Part model, mm, in its own coordinate system. A direction names the side the tool comes from. Coordinates: 2 decimals unless noted, no trailing zeros. Loops run counter-clockwise (first coordinate to the right, second up) from the corner with the lowest first, then second, coordinate; pieces in that order, holes last. Notation, with made-up numbers: (86, 78) -> (104, 78) arc R19 ccw to (104, 96) -> close; hole circle Ø4 at (80, 89). An arc over 180 degrees is marked (long way). Use one line per item in the form item = value. Start each with the question number.
(1) Pin check, flat tips, straight feed: P1, Ø5, axis at y = 5, z = -50, coming from the +X side; P2, Ø5, axis at y = 5.5, z = -41, coming from the -X side; P3, Ø2.5, axis at x = 0, z = 0.5, coming from the -Y side; P4, Ø2.5, axis at x = -17, z = 0, coming from the +Y side. Stop position of each tip, or through.
(2) Band-saw the part on A-A on x = 48. Give the cut face in (y, z), then the cut area to 3 significant figures.
(3) Mould opens along X. For faces 1 (the flat face through (-1, 9, 1)), 2 (the flat face through (-35.275, 3.042, -20.366)), 3 (the cylindrical face through (-0.652, 3.042, 5.964)) say: +X half, -X half, draft (parallel to the pull), parting line (faces both ways), or undercut.
(4) Drill centre lines: L1, parallel to X at y = 7.2, z = 0; L2, parallel to Y at x = -30, z = -43. Where is each one in solid material? Low to high. Write a range as [from, to].
(5) Band-saw the part on B-B on z = 24. Give the cut face in (x, y).
(6) 3-axis set-ups, long thin cutter, end or side, ignore diameter. For faces 4 (the flat face through (33.263, 3.042, 24.176)), 5 (the flat face through (-24.176, 3.042, 33.263)), 6 (the cylindrical face through (5.964, 3.042, 0.652)), 7 (the cylindrical face through (0.652, 3.042, -5.964)), 8 (the flat face through (0, 6, 0)): which of +Z, -Z, +X, -X, +Y, -Y reach the whole face in a straight line?
Autodesk Inventor part; units mm, degrees
ref_plane "YZ Plane" through (0, 0, 0) normal (1, 0, 0) x (0, 1, 0)
ref_plane "XZ Plane" through (0, 0, 0) normal (0, 1, 0) x (-1, 0, 0)
ref_plane "XY Plane" through (0, 0, 0) normal (0, 0, 1) x (1, 0, 0)
sketch "Sketch1" plane through (0, 0, 0) normal (0, 0, 1) x (1, 0, 0)
  line L0 (4, 0) -> (6, 0)
  line L1 (6, 0) -> (6, 6)
  line L2 (6, 6) -> (76.45, 6)
  line L3 (76.45, 6) -> (76.45, 9)
  line L4 (4, 6) -> (4, 0)
  line L5 (0, 9) -> (0, 6)
  line L6 (0, 6) -> (4, 6)
  line L7 (0, 9) -> (13.95, 9)
  line L8 (13.95, 9) -> (13.95, 9)
  line L9 (13.95, 9) -> (16.45, 9)
  line L10 (16.45, 9) -> (16.45, 9)
  line L11 (16.45, 9) -> (76.45, 9)
  point P0 (0, 0)
  dimension "d0" = 4
  dimension "d1" = 6
  dimension "d2" = 0
  dimension "d3" = 3
  dimension "d4" = 2
  dimension "d7" = 2.5
  dimension "d8" = 60
  dimension "d9" = 13.95
  dimension "d10" = 0
revolve "Revolution1" add sketch "Sketch1" angle 360 about axis through (0, 9, 0) along (0, -1, 0)
thread "Thread1"
sketch "Sketch2" plane through (0, 9, 0) normal (0, 1, 0) x (1, 0, 0)
  circle A0 centre (17, 0) radius 1.6
  circle A1 centre (-17, 0) radius 1.6
  circle A2 centre (0, 17) radius 1.6
  circle A3 centre (0, -17) radius 1.6
  point P0 (0, 0)
  dimension "d14" = 3.2
  dimension "d15" = 3.2
  dimension "d16" = 3.2
  dimension "d17" = 3.2
  dimension "d18" = 34
  dimension "d19" = 17
  dimension "d20" = 34
  dimension "d21" = 17
extrude "Extrusion1" cut sketch "Sketch2" against normal through all
sketch "Sketch5" plane through (0, 6, 0) normal (0, -1, 0) x (1, 0, 0)
  circle A0 centre (0, 0) radius 76.45
  circle A1 centre (0, 0) radius 6
  circle A2 centre (0, 0) radius 4
  line L0 (-5.1962, -3) -> (-66.2076, -38.225)
  line L1 (-63.7866, -42.1411) -> (-1.873, -5.7002)
  line L2 (42.1411, -63.7866) -> (5.7002, -1.873)
  line L3 (3, -5.1962) -> (38.225, -66.2076)
  line L4 (63.7866, 42.1411) -> (1.873, 5.7002)
  line L5 (5.1962, 3) -> (66.2076, 38.225)
  line L6 (-42.1411, 63.7866) -> (-5.7002, 1.873)
  line L7 (-3, 5.1962) -> (-38.225, 66.2076)
  arc A3 (38.225, -66.2076) -> (42.1411, -63.7866) centre (0, 0) ccw
  arc A4 (66.2076, 38.225) -> (63.7866, 42.1411) centre (0, 0) ccw
  arc A5 (-38.225, 66.2076) -> (-42.1411, 63.7866) centre (0, 0) ccw
  arc A6 (-66.2076, -38.225) -> (-63.7866, -42.1411) centre (0, 0) ccw
  arc A7 (-5.1962, -3) -> (-1.873, -5.7002) centre (0, 0) ccw
  arc A8 (-3, 5.1962) -> (-5.7002, 1.873) centre (0, 0) ccw
  arc A9 (3, -5.1962) -> (5.7002, -1.873) centre (0, 0) ccw
  arc A10 (5.1962, 3) -> (1.873, 5.7002) centre (0, 0) ccw
  point P0 (0, 0)
  point P1 (-38.225, 66.2076)
  point P2 (-42.1411, 63.7866)
  point P3 (-5.7002, 1.873)
  point P4 (5.1962, 3)
  point P5 (66.2076, 38.225)
  point P6 (63.7866, 42.1411)
  point P7 (1.873, 5.7002)
  point P8 (38.225, -66.2076)
  point P9 (42.1411, -63.7866)
  point P10 (5.7002, -1.873)
  dimension "d35" = 360
extrude "Extrusion3" add sketch "Sketch5" along normal blind 6 contours L5 A1 L4 A0 | A0 L3 A1 L2 | L7 A1 L6 A0 | A0 L0 A1 L1
properties part number "motor platform reaction wheel" material "ABS Plastic"
A:
q1.P1 = 59.74
q1.P2 = -66.05
q1.P3 = 6
q1.P4 = through
q2.outline = (0, 27.71) -> (6, 27.71) -> (6, -59.5) -> (9, -59.5) -> (9, 59.5) -> (6, 59.5) -> (6, 32.85) -> (0, 32.85) -> close
q2.area = 388 mm²
q3.face_1 = draft
q3.face_2 = -X half
q3.face_3 = undercut
q4.L1 = [-76.45, -18.6], [-15.4, 15.4], [18.6, 76.45]
q4.L2 = [6, 9]
q5.outline = (-72.59, 6) -> (-18.72, 6) -> (-18.72, 0) -> (-13.86, 0) -> (-13.86, 6) -> (32.96, 6) -> (32.96, 0) -> (41.57, 0) -> (41.57, 6) -> (72.59, 6) -> (72.59, 9) -> (-72.59, 9) -> close
q6.face_4 = +Z, -Y
q6.face_5 = -X, -Y
q6.face_6 = +X, -Y
q6.face_7 = -Z, -Y
q6.face_8 = -Y
